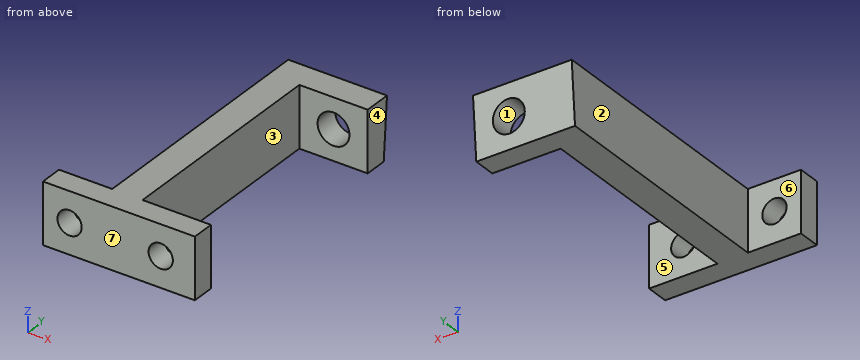
from build123d import *

# Parameters (mm, degrees)
SKETCH1_W             = 8.012892266
SKETCH1_H             = 3
BOSS_EXTRUDE1_DEPTH   = 9
BOSS_EXTRUDE1_2_DEPTH = 9
BOSS_EXTRUDE2_START   = -9
BOSS_EXTRUDE2_DEPTH   = 4
BOSS_EXTRUDE3_START   = -13
SKETCH1_4_W           = 8.012892266
SKETCH1_4_H           = 3
BOSS_EXTRUDE3_DEPTH   = 7
CUT_EXTRUDE1_REACH    = 136.557
SKETCH2_R             = 1.6
CUT_EXTRUDE2_REACH    = 136.408
SKETCH3_R             = 2.1


with BuildPart() as part:
    # Sketch1 → Boss-Extrude1 (new body)
    with BuildSketch(Plane(origin=(-20.116663772, 0, 0), x_dir=(0, 0, -1), z_dir=(1, 0, 0))):
        with Locations((120.127472222, 75.181369419)):
            Rectangle(SKETCH1_W, SKETCH1_H)
    extrude(amount=-BOSS_EXTRUDE1_DEPTH)



with BuildPart() as body_2:
    # Sketch1 → Boss-Extrude1 2 (new body)
    with BuildSketch(Plane(origin=(-20.116663772, 0, 0), x_dir=(0, 0, -1), z_dir=(1, 0, 0))):
        Polygon((116.121026089, 106.035971289), (124.133918355, 106.035971289), (124.133918355, 109.035971289), (116.121026089, 109.651271917), align=None)
    extrude(amount=-BOSS_EXTRUDE1_2_DEPTH)


with BuildPart() as part_1:
    add(part.part)

    add(body_2.part)  # Boss-Extrude2 merges body 2
    # Sketch1<3> → Boss-Extrude2 (add)
    with BuildSketch(Plane(origin=(-20.116663772, 0, 0), x_dir=(0, 0, -1), z_dir=(1, 0, 0)).offset(BOSS_EXTRUDE2_START)):
        Polygon((116.121026089, 73.681369419), (124.133918355, 73.681369419), (124.133918355, 109.035971289), (116.121026089, 109.651271917), align=None)
    extrude(amount=-BOSS_EXTRUDE2_DEPTH)

    # Sketch1<4> → Boss-Extrude3 (add)
    with BuildSketch(Plane(origin=(-20.116663772, 0, 0), x_dir=(0, 0, -1), z_dir=(1, 0, 0)).offset(BOSS_EXTRUDE3_START)):
        with Locations((120.127472222, 75.181369419)):
            Rectangle(SKETCH1_4_W, SKETCH1_4_H)
    extrude(amount=-BOSS_EXTRUDE3_DEPTH)

    # Sketch2 → Cut-Extrude1 (cut, up to next)
    with BuildSketch(Plane(origin=(0, 76.681369419, 0), x_dir=(1, 0, 0), z_dir=(0, 1, 0)), mode=Mode.PRIVATE) as cut_extrude1_sk1:
        with Locations(Location((-24.616663772, 120.127472222, 0), (0, 0, 180))):
            Circle(SKETCH2_R)
    cut_extrude1_tool1 = extrude(cut_extrude1_sk1.sketch, amount=-CUT_EXTRUDE1_REACH, mode=Mode.PRIVATE) & part_1.part
    # Sketch2 → Cut-Extrude1 (cut, up to next)
    with BuildSketch(Plane(origin=(0, 76.681369419, 0), x_dir=(1, 0, 0), z_dir=(0, 1, 0)), mode=Mode.PRIVATE) as cut_extrude1_sk2:
        with Locations(Location((-36.616663772, 120.127472222, 0), (0, 0, 180))):
            Circle(SKETCH2_R)
    cut_extrude1_tool2 = extrude(cut_extrude1_sk2.sketch, amount=-CUT_EXTRUDE1_REACH, mode=Mode.PRIVATE) & part_1.part
    add(cut_extrude1_tool1.solids().sort_by_distance((-24.616664, 76.681369, -120.127472))[0], mode=Mode.SUBTRACT)
    add(cut_extrude1_tool2.solids().sort_by_distance((-36.616664, 76.681369, -120.127472))[0], mode=Mode.SUBTRACT)

    # Cut-Extrude2: up to this plane
    cut_extrude2_end = Plane(origin=(-33.116663772, 117.873028528, -9.051332034), z_dir=(1.1764260283030438e-15, -0.9970647123754436, 0.07656343341095784))
    # Sketch3 → Cut-Extrude2 (cut, up to the surface)
    with BuildSketch(Plane.XZ.offset(-106.035971289), mode=Mode.PRIVATE) as cut_extrude2_sk1:
        with Locations((-24.616663772, -120.127472222)):
            Circle(SKETCH3_R)
    cut_extrude2_tool1 = split(extrude(cut_extrude2_sk1.sketch, amount=-CUT_EXTRUDE2_REACH, mode=Mode.PRIVATE), bisect_by=cut_extrude2_end, keep=Keep.BOTH, mode=Mode.PRIVATE)
    add(cut_extrude2_tool1.solids().sort_by_distance((-24.616664, 106.035971, -120.127472))[0], mode=Mode.SUBTRACT)


solid = part_1.part
Could you check a few things on this model? Use its own coordinates, in mm. Face numbers are marked on the shaded views. A direction names the side the tool comes from. Round coordinates to 2 decimals unless told otherwise and drop trailing zeros. Write each loop counter-clockwise with the first axis right and the second up, starting at its lowest first coordinate (ties: lowest second). Pieces come first, ordered by that corner, then holes. Notation, with made-up numbers: (86, -37.75) - (126, -37.75) arc R18 ccw to (126, -7.75) - close; hole circle Ø5 at (-18, 35). An arc over 180 degrees is marked (long way). Put each result on its own line as item: value. Start each with the question number.
(1) Will these pins go through, and if not, where does the flat tip stop? pin 1 (4 mm diameter, centred on x = -36.62, z = -120.13, fed in from +Y); pin 2 (4 mm diameter, centred on y = 100.5, z = -118.5, fed in from +X); pin 3 (4 mm diameter, centred on y = 98.5, z = -122, fed in from -X).
(2) I want a section at D-D, the plane y = 101.5. Please give me the cut outline in (x, z), plus the area to 3 significant figures.
(3) I want a section at C-C, the plane z = -119.25. Please give me the cut outline in (x, y), plus the area to 3 significant figures.
(4) I want a section at A-A, the plane x = -28.75. Please give me the cut outline in (y, z).
(5) Thinking about a two-plate mould opening in Y: for the marked faces 5, 6 and 7, which applies, released by +Y, released by -Y, zero draft, split by the parting line, or undercut?
(6) I want a section at B-B, the plane x = -25. Please give me the cut outline in (y, z), plus the area to 3 significant figures.
(7) For the marked faces 1, 2, 3 and 4, which set-ups out of +Z, -Z, +X, -X, +Y, -Y let a thin tool reach every point of the face, with its end or its side?
(8) I need wall thicknesses on probe 1 along Y at (x, z) = (-21.25, -118); probe 2 along Y at (x, z) = (-36, -122); probe 3 along X at (y, z) = (83.5, -120.25). Which ranges of each line are inside material? Lowest first, please.
Here are the results:
1. pin 1: stops at y = 76.68
1. pin 2: stops at x = -29.12
1. pin 3: stops at x = -33.12
2. outline: (-33.12, -124.13) - (-29.12, -124.13) - (-29.12, -116.12) - (-33.12, -116.12) - close
2. area: 32.1 mm^2
3. outline: (-40.12, 73.68) - (-37.95, 73.68) - (-37.95, 76.68) - (-40.12, 76.68) - close; (-35.28, 73.68) - (-25.95, 73.68) - (-25.95, 76.68) - (-29.12, 76.68) - (-29.12, 106.04) - (-26.52, 106.04) - (-26.52, 109.41) - (-33.12, 109.41) - (-33.12, 76.68) - (-35.28, 76.68) - close; (-23.28, 73.68) - (-20.12, 73.68) - (-20.12, 76.68) - (-23.28, 76.68) - close; (-22.71, 106.04) - (-20.12, 106.04) - (-20.12, 109.41) - (-22.71, 109.41) - close
3. area: 192 mm^2
4. outline: (73.68, -124.13) - (76.68, -124.13) - (76.68, -116.12) - (73.68, -116.12) - close; (106.04, -124.13) - (109.04, -124.13) - (109.65, -116.12) - (106.04, -116.12) - close
5. face 5: undercut
5. face 6: released by +Y
5. face 7: released by -Y
6. outline: (73.68, -124.13) - (76.68, -124.13) - (76.68, -121.68) - (73.68, -121.68) - close; (73.68, -118.57) - (76.68, -118.57) - (76.68, -116.12) - (73.68, -116.12) - close; (106.04, -124.13) - (109.04, -124.13) - (109.19, -122.19) - (106.04, -122.19) - close; (106.04, -118.06) - (109.5, -118.06) - (109.65, -116.12) - (106.04, -116.12) - close
6. area: 27.6 mm^2
7. face 1: +Y
7. face 2: +Z, -Z, -X, +Y
7. face 3: +Z, -Z, +X
7. face 4: +Z, -Z, +X, +Y, -Y
8. probe 1: y = 73.68 to 76.68, 106.04 to 109.51
8. probe 2: y = 73.68 to 76.68
8. probe 3: x = -33.12 to -29.12
